Could you check a few things on this model? Use its own coordinates, in mm. Coordinates: 2 decimals unless noted, no trailing zeros. Loops run counter-clockwise (first coordinate to the right, second up) from the corner with the lowest first, then second, coordinate; pieces in that order, holes last.
from build123d import *

# Parameters (mm, degrees)
SKETCH1_W           = 115
SKETCH1_H           = 100
SKETCH1_R           = 6
BOSS_EXTRUDE2_DEPTH = 10
FILLET1_R           = 5


with BuildPart() as part:
    # Sketch1 → Boss-Extrude2 (new body)
    with BuildSketch(Plane(origin=(0, 0, 0), x_dir=(1, 0, 0), z_dir=(0, 1, 0))):
        Rectangle(SKETCH1_W, SKETCH1_H)
        with Locations(Location((-46, 38, 0), (0, 0, 270))):
            Circle(SKETCH1_R, mode=Mode.SUBTRACT)
        with Locations(Location((46, 38, 0), (0, 0, 270))):
            Circle(SKETCH1_R, mode=Mode.SUBTRACT)
        with Locations(Location((46, -38, 0), (0, 0, 270))):
            Circle(SKETCH1_R, mode=Mode.SUBTRACT)
        with Locations(Location((-46, -38, 0), (0, 0, 270))):
            Circle(SKETCH1_R, mode=Mode.SUBTRACT)
        with Locations(Location((0, 0, 0), (0, 0, 270))):
            Circle(SKETCH1_R, mode=Mode.SUBTRACT)
    extrude(amount=BOSS_EXTRUDE2_DEPTH)

    # Fillet1
    fillet1_edges = [part.edges().sort_by_distance(p)[0] for p in [
        (-57.5, 5, -50),
        (57.5, 5, -50),
        (57.5, 5, 50),
        (-57.5, 5, 50),
    ]]
    fillet(fillet1_edges, radius=FILLET1_R)


solid = part.part
1) Imagine slicing it at D-D on z = 0. List the corners of the cut face in (x, y) for me, plus the area to 3 significant figures.
2) Imagine slicing it at A-A on x = 46. List the corners of the cut face in (y, z) for me.
3) Will this pin go through, and if not, where does the flat tip stop? pin 1 (11 mm diameter, centred on x = -46, z = 38, fed in from +Y).
4) Imagine slicing it at B-B on z = 38. List the corners of the cut face in (x, y) for me.
5) If I drill on L1, parallel to Z at x = 45.5, y = 6; L2, parallel to X at y = 2.75, z = 38; L3, parallel to X at y = 6, z = -42, over which ranges is the centre line in solid material (lowest first)?
6) We'd pull the mould along Z, two halves only. Please class faces 1 (the flat face through (57.5, 5, 1)), 2 (the cylindrical face through (-56.07, 5.07, 48.5)), 3 (the cylindrical face through (-49.65, 4.93, -42.76)): released by +Z, released by -Z, zero draft, split by the parting line, or undercut.
7) Imagine slicing it at C-C on y = 1.25. List the corners of the cut face in (x, z) for me.
Solved:
1. outline: (-57.5, 0) - (-6, 0) - (-6, 10) - (-57.5, 10) - close; (6, 0) - (57.5, 0) - (57.5, 10) - (6, 10) - close
1. area: 1,030 mm2
2. outline: (0, -50) - (10, -50) - (10, -44) - (0, -44) - close; (0, -32) - (10, -32) - (10, 32) - (0, 32) - close; (0, 44) - (10, 44) - (10, 50) - (0, 50) - close
3. pin 1: passes through
4. outline: (-57.5, 0) - (-52, 0) - (-52, 10) - (-57.5, 10) - close; (-40, 0) - (40, 0) - (40, 10) - (-40, 10) - close; (52, 0) - (57.5, 0) - (57.5, 10) - (52, 10) - close
5. L1: z = -50 to -43.98, -32.02 to 32.02, 43.98 to 50
5. L2: x = -57.5 to -52, -40 to 40, 52 to 57.5
5. L3: x = -57.5 to -50.47, -41.53 to 41.53, 50.47 to 57.5
6. face 1: zero draft
6. face 2: released by +Z
6. face 3: undercut
7. outline: (-57.5, -45) arc R5 ccw to (-52.5, -50) - (52.5, -50) arc R5 ccw to (57.5, -45) - (57.5, 45) arc R5 ccw to (52.5, 50) - (-52.5, 50) arc R5 ccw to (-57.5, 45) - close; hole circle Ø12 at (-46, -38); hole circle Ø12 at (-46, 38); hole circle Ø12 at (0, 0); hole circle Ø12 at (46, -38); hole circle Ø12 at (46, 38)
